The model under review builds one solid part; all positions refer to its coordinate system, in mm. A direction names the side the tool comes from. Give positions to 0.01 mm unless a question says otherwise; leave off trailing zeros. Loops run counter-clockwise (first coordinate to the right, second up) from the corner with the lowest first, then second, coordinate; pieces in that order, holes last. Notation, with made-up numbers: (83, -37) - (132, -37) arc R23 ccw to (132, -4) - close; hole circle Ø6 at (55.5, 62.5). An arc over 180 degrees is marked (long way). Return JSON: item names as keys, results as strings. Group by question number.
```python
from build123d import *

# Parameters (mm, degrees)
ARM_WEB_START               = 8
PROFILE_1_R                 = 5.05
PROFILE_1_R_2               = 1.65
ARM_WEB_DEPTH               = 10
PROFILE_2_R                 = 17.2
PROFILE_2_R_2               = 5
PROFILE_2_R_3               = 1.65
ROTOR_STANDOFF_DEPTH        = 8
ROTOR_SCREW_SPOTFACES_START = 12
PROFILE_3_R                 = 3
ROTOR_SCREW_SPOTFACES_DEPTH = 6.01


with BuildPart() as part:
    # Profile_1 → Arm_web (new body)
    with BuildSketch(Plane.XY.offset(ARM_WEB_START)):
        Polygon((-116.111272563, 9.146165735), (-119.146165735, 6.111272563), (-120.788638084, 2.145993542), (-120.788638084, -2.145993542), (-119.146165735, -6.111272563), (-116.111272563, -9.146165735), (-112.145993542, -10.788638084), (-3.706716118, -18.634920328), (3.706716118, -18.634920328), (10.555834427, -15.797922634), (15.797922634, -10.555834427), (18.634920328, -3.706716118), (18.634920328, 3.706716118), (15.797922634, 10.555834427), (10.555834427, 15.797922634), (3.706716118, 18.634920328), (-3.706716118, 18.634920328), (-112.145993542, 10.788638084), align=None)
        with Locations((-110, 0)):
            Circle(PROFILE_1_R, mode=Mode.SUBTRACT)
        with Locations((-13.5, 0)):
            Circle(PROFILE_1_R_2, mode=Mode.SUBTRACT)
        with Locations((-6.75, 11.691342951)):
            Circle(PROFILE_1_R_2, mode=Mode.SUBTRACT)
        with Locations((6.75, 11.691342951)):
            Circle(PROFILE_1_R_2, mode=Mode.SUBTRACT)
        with Locations((13.5, 0)):
            Circle(PROFILE_1_R_2, mode=Mode.SUBTRACT)
        with Locations((6.75, -11.691342951)):
            Circle(PROFILE_1_R_2, mode=Mode.SUBTRACT)
        with Locations((-6.75, -11.691342951)):
            Circle(PROFILE_1_R_2, mode=Mode.SUBTRACT)
    extrude(amount=ARM_WEB_DEPTH)

    # Profile_2 → Rotor_standoff (add)
    with BuildSketch(Plane.XY):
        Circle(PROFILE_2_R)
        Circle(PROFILE_2_R_2, mode=Mode.SUBTRACT)
        with Locations((-13.5, 0)):
            Circle(PROFILE_2_R_3, mode=Mode.SUBTRACT)
        with Locations((-6.75, 11.691342951)):
            Circle(PROFILE_2_R_3, mode=Mode.SUBTRACT)
        with Locations((6.75, 11.691342951)):
            Circle(PROFILE_2_R_3, mode=Mode.SUBTRACT)
        with Locations((13.5, 0)):
            Circle(PROFILE_2_R_3, mode=Mode.SUBTRACT)
        with Locations((6.75, -11.691342951)):
            Circle(PROFILE_2_R_3, mode=Mode.SUBTRACT)
        with Locations((-6.75, -11.691342951)):
            Circle(PROFILE_2_R_3, mode=Mode.SUBTRACT)
    extrude(amount=ROTOR_STANDOFF_DEPTH)

    # Profile_3 → Rotor_screw_spotfaces (cut)
    with BuildSketch(Plane.XY.offset(ROTOR_SCREW_SPOTFACES_START)):
        with Locations(Location((-13.5, 0, 0), (0, 0, 180))):
            Circle(PROFILE_3_R)
        with Locations(Location((-6.75, 11.691342951, 0), (0, 0, 180))):
            Circle(PROFILE_3_R)
        with Locations(Location((6.75, 11.691342951, 0), (0, 0, 180))):
            Circle(PROFILE_3_R)
        with Locations(Location((13.5, 0, 0), (0, 0, 180))):
            Circle(PROFILE_3_R)
        with Locations(Location((6.75, -11.691342951, 0), (0, 0, 180))):
            Circle(PROFILE_3_R)
        with Locations(Location((-6.75, -11.691342951, 0), (0, 0, 180))):
            Circle(PROFILE_3_R)
    extrude(amount=ROTOR_SCREW_SPOTFACES_DEPTH, mode=Mode.SUBTRACT)


solid = part.part
```
1) Tool access review of faces 4 (the face through (0, -18.635, 13)), 5 (the face through (-10.5, -0.1, 15)): name each direction out of +Z, -Z, +X, -X, +Y, -Y from which nothing blocks a thin tool from reaching the whole face with its end or side.
2) Draft analysis for pull direction X (two halves, no side actions). For faces 1 (the face through (-7.11, 10.08, 5.92)), 2 (the face through (4, -4, 0)), 3 (the face through (-114.156, -9.956, 12.93)), state which applies: +X half, -X half, draft (parallel to the pull), parting line (faces both ways), or undercut.
3) We need section B-B, the plane z = 13.25. Write out the cut boundary in (x, y), plus the area to 3 significant figures.
4) We need section C-C, the plane x = -6.75. Write out the cut boundary in (y, z), plus the area to 3 significant figures.
5) For pin 1 Ø3 at (y, z) = (4, 6) entering from +X; pin 2 Ø2 at (x, z) = (-60.5, 10) entering from -Y; pin 3 Ø2 at (x, y) = (-23, 14) entering from -Z; pin 4 Ø2 at (x, y) = (-6.75, -11.69) entering from -Z, all flat-tipped, find the tip position at first contact; note any pin that passes through.
6) We need section D-D, the plane z = 4.5. Write out the cut boundary in (x, y), plus the area to 3 significant figures.
7) We need section A-A, the plane x = 13.5. Write out the cut boundary in (y, z).
8) To check wall thickness, follow line 1 (Y direction, x = -6.75, z = 6); line 2 (X direction, y = -2, z = 16.5); line 3 (X direction, y = -13, z = 6.75). State the ranges of each line that lie inside material, in increasing order.
Findings:
{
 "1": {"face 4": "+Z, -Z, +X, -X, -Y", "face 5": "+Z"},
 "2": {"face 1": "undercut", "face 2": "draft", "face 3": "-X half"},
 "3": {"outline": "(-120.79, -2.15) - (-119.15, -6.11) - (-116.11, -9.15) - (-112.15, -10.79) - (-3.71, -18.63) - (3.71, -18.63) - (10.56, -15.8) - (15.8, -10.56) - (18.63, -3.71) - (18.63, 3.71) - (15.8, 10.56) - (10.56, 15.8) - (3.71, 18.63) - (-3.71, 18.63) - (-112.15, 10.79) - (-116.11, 9.15) - (-119.15, 6.11) - (-120.79, 2.15) - close; hole circle Ø10.1 at (-110, 0); hole circle Ø6 at (-13.5, 0); hole circle Ø6 at (-6.75, -11.69); hole circle Ø6 at (-6.75, 11.69); hole circle Ø6 at (6.75, -11.69); hole circle Ø6 at (6.75, 11.69); hole circle Ø6 at (13.5, 0)", "area": "3,770 mm^2"},
 "4": {"outline": "(-18.41, 8) - (-15.82, 8) - (-15.82, 0) - (-13.34, 0) - (-13.34, 12) - (-14.69, 12) - (-14.69, 18) - (-18.41, 18) - close; (-10.04, 0) - (10.04, 0) - (10.04, 12) - (8.69, 12) - (8.69, 18) - (-8.69, 18) - (-8.69, 12) - (-10.04, 12) - close; (13.34, 0) - (15.82, 0) - (15.82, 8) - (18.41, 8) - (18.41, 18) - (14.69, 18) - (14.69, 12) - (13.34, 12) - close", "area": "470 mm^2"},
 "5": {"pin 1": "stops at x = 17.02", "pin 2": "stops at y = -14.6", "pin 3": "stops at z = 8", "pin 4": "passes through"},
 "6": {"outline": "circle Ø34.4 at (0, 0); hole circle Ø3.3 at (-13.5, 0); hole circle Ø3.3 at (-6.75, -11.69); hole circle Ø3.3 at (-6.75, 11.69); hole circle Ø10 at (0, 0); hole circle Ø3.3 at (6.75, -11.69); hole circle Ø3.3 at (6.75, 11.69); hole circle Ø3.3 at (13.5, 0)", "area": "800 mm^2"},
 "7": {"outline": "(-12.85, 8) - (-10.66, 8) - (-10.66, 0) - (-1.65, 0) - (-1.65, 12) - (-3, 12) - (-3, 18) - (-12.85, 18) - close; (1.65, 0) - (10.66, 0) - (10.66, 8) - (12.85, 8) - (12.85, 18) - (3, 18) - (3, 12) - (1.65, 12) - close"},
 "8": {"line 1": "y = -15.82 to -13.34, -10.04 to 10.04, 13.34 to 15.82", "line 2": "x = -120.79 to -114.64, -105.36 to -15.74, -11.26 to 11.26, 15.74 to 18.63", "line 3": "x = -11.26 to -7.75, -5.75 to 5.75, 7.75 to 11.26"}
}
